Model file for the job. Use its own axes, mm. A direction names the side the tool comes from. Round coordinates to 2 decimals unless told otherwise and drop trailing zeros. Write each loop counter-clockwise with the first axis right and the second up, starting at its lowest first coordinate (ties: lowest second). Pieces come first, ordered by that corner, then holes. Notation, with made-up numbers: (39.5, 61.5) - (98.5, 61.5) arc R27 cw to (98.5, 94.5) - close; hole circle Ø2 at (-12, 11). An arc over 180 degrees is marked (long way). One line per item, written item: value.
from build123d import *

# Parameters (mm, degrees)
SKETCH1_W           = 25
SKETCH1_H           = 25
BOSS_EXTRUDE1_DEPTH = 6
BOSS_EXTRUDE3_DEPTH = 4
SKETCH2_R           = 2.25
CUT_EXTRUDE1_DEPTH  = 6
SKETCH9_W           = 25
SKETCH9_H           = 6
CUT_EXTRUDE2_DEPTH  = 1
SKETCH11_W          = 36.82832664
SKETCH11_H          = 4
BOSS_EXTRUDE4_DEPTH = 20
SKETCH13_R          = 2.1
CUT_EXTRUDE3_DEPTH  = 50.410927182
FILLET2_R           = 10
CHAMFER1_SIZE       = 0.75
CHAMFER2_SIZE       = 0.75
CHAMFER3_SIZE       = 0.75


with BuildPart() as part:
    # Sketch1 → Boss-Extrude1 (new body)
    with BuildSketch(Plane(origin=(0, 0, 0), x_dir=(1, 0, 0), z_dir=(0, 1, 0))):
        with Locations((12.5, 12.5)):
            Rectangle(SKETCH1_W, SKETCH1_H)
    extrude(amount=BOSS_EXTRUDE1_DEPTH)

    # Sketch5 → Boss-Extrude3 (add)
    with BuildSketch(Plane.XY):
        Polygon((-5.91332664, 12.95), (30.915, 12.95), (30, -5.62), (-5, -5.62), align=None)
    extrude(amount=-BOSS_EXTRUDE3_DEPTH)

    # Sketch2 → Cut-Extrude1 (cut)
    with BuildSketch(Plane.XZ):
        with Locations(Location((5.5, -16, 0), (0, 0, 270))):
            Circle(SKETCH2_R)
        with Locations(Location((19.5, -16, 0), (0, 0, 90))):
            Circle(SKETCH2_R)
    extrude(amount=-CUT_EXTRUDE1_DEPTH, mode=Mode.SUBTRACT)

    # Sketch9 → Cut-Extrude2 (cut)
    with BuildSketch(Plane(origin=(0, 0, -25), x_dir=(-1, 0, 0), z_dir=(0, 0, -1))):
        with Locations((-12.5, 3)):
            Rectangle(SKETCH9_W, SKETCH9_H)
    extrude(amount=-CUT_EXTRUDE2_DEPTH, mode=Mode.SUBTRACT)

    # Sketch11 → Boss-Extrude4 (add)
    with BuildSketch(Plane(origin=(0, 12.95, 0), x_dir=(1, 0, 0), z_dir=(0, 1, 0))):
        with Locations((12.50083668, 2)):
            Rectangle(SKETCH11_W, SKETCH11_H)
    extrude(amount=BOSS_EXTRUDE4_DEPTH)

    # Sketch13 → Cut-Extrude3 (cut, through all)
    with BuildSketch(Plane(origin=(0, 0, -4), x_dir=(-1, 0, 0), z_dir=(0, 0, -1))):
        with Locations((-21.25, 26)):
            Circle(SKETCH13_R)
        with Locations((-3.75, 26)):
            Circle(SKETCH13_R)
    extrude(amount=-CUT_EXTRUDE3_DEPTH, mode=Mode.SUBTRACT)

    # Fillet2
    fillet2_edges = [part.edges().sort_by_distance(p)[0] for p in [
        (30, -5.62, -2),
        (-5, -5.62, -2),
        (-5.91332664, 32.95, -2),
        (30.915, 32.95, -2),
    ]]
    fillet(fillet2_edges, radius=FILLET2_R)

    # Chamfer1
    # the kernel refuses this chamfer: 0.75 mm, written as the material it takes off along each edge
    with BuildSketch(Plane(origin=(20.480598416, -5.62, 0), x_dir=(0, 0.9996219169112968, 0.02749587661058636), z_dir=(-1, 0, 0)), Plane(origin=(20.480598416, -5.62, -4), x_dir=(0, -0.02749587661058678, 0.9996219169112968), z_dir=(-1, 0, 0))) as chamfer1_piece_1:
        Polygon((CHAMFER1_SIZE * 0.999621916911, CHAMFER1_SIZE * 0.0274958766106), (-CHAMFER1_SIZE * 0.0274958766106, CHAMFER1_SIZE * 0.999621916911), (0, 0), align=None)
    extrude(amount=15.960340029, mode=Mode.SUBTRACT)
    with BuildSketch(Plane(origin=(31.009920786, 14.876425142, 0), x_dir=(-0.9984106656617833, 0.04919470969738991, 0.027495876610586206), z_dir=(-0.04921331642006734, -0.9987882906236629, 0)), Plane(origin=(31.009920786, 14.876425142, -4), x_dir=(0.027462559599087527, -0.0013531632758839558, 0.9996219169112968), z_dir=(-0.04921331642006734, -0.9987882906236629, 0))) as chamfer1_piece_2:
        Polygon((CHAMFER1_SIZE * 0.999621916911, CHAMFER1_SIZE * 0.0274958766106), (-CHAMFER1_SIZE * 0.0274958766106, CHAMFER1_SIZE * 0.999621916911), (0, 0), align=None)
    extrude(amount=11.001889398, mode=Mode.SUBTRACT)
    with BuildSketch(Plane(origin=(30.915, 11.021237759, 0), x_dir=(-0.9996219169112968, 0, 0.02749587661058636), z_dir=(0, 1, 0)), Plane(origin=(30.915, 11.021237759, -4), x_dir=(0.02749587661058678, 0, 0.9996219169112968), z_dir=(0, 1, 0))) as chamfer1_piece_3:
        Polygon((CHAMFER1_SIZE * 0.999621916911, -CHAMFER1_SIZE * 0.0274958766106), (-CHAMFER1_SIZE * 0.0274958766106, -CHAMFER1_SIZE * 0.999621916911), (0, 0), align=None)
    extrude(amount=11.928762241, mode=Mode.SUBTRACT)
    with BuildSketch(Plane(origin=(4.08667336, 32.95, 0), x_dir=(0, -0.9996219169112968, 0.027495876610586487), z_dir=(1, 0, 0))) as chamfer1_piece_4:
        Polygon((CHAMFER1_SIZE * 0.999621916911, CHAMFER1_SIZE * 0.0274958766106), (-CHAMFER1_SIZE * 0.0274958766106, CHAMFER1_SIZE * 0.999621916911), (0, 0), align=None)
    extrude(amount=16.82832664, mode=Mode.SUBTRACT)
    with BuildSketch(Plane(origin=(-5.91332664, 11.021237759, 0), x_dir=(0.9996219169112968, 0, 0.02749587661058636), z_dir=(0, 1, 0)), Plane(origin=(-5.91332664, 11.021237759, -4), x_dir=(-0.02749587661058678, 0, 0.9996219169112968), z_dir=(0, 1, 0))) as chamfer1_piece_5:
        Polygon((CHAMFER1_SIZE * 0.999621916911, CHAMFER1_SIZE * 0.0274958766106), (-CHAMFER1_SIZE * 0.0274958766106, CHAMFER1_SIZE * 0.999621916911), (0, 0), align=None)
    extrude(amount=11.928762241, mode=Mode.SUBTRACT)
    with BuildSketch(Plane(origin=(20.915, 22.95, 0), x_dir=(1, 0, 0), z_dir=(0, -1, 0))) as chamfer1_piece_6:
        Polygon((10 - CHAMFER1_SIZE, 0), (10, -CHAMFER1_SIZE), (10, 0), align=None)
    revolve(axis=Axis((20.915, 22.95, 0), (0, 0, 1)), revolution_arc=90, mode=Mode.SUBTRACT)
    with BuildSketch(Plane(origin=(4.08667336, 22.95, 0), x_dir=(0, 1, 0), z_dir=(1, 0, 0))) as chamfer1_piece_7:
        Polygon((10 - CHAMFER1_SIZE, 0), (10, -CHAMFER1_SIZE), (10, 0), align=None)
    revolve(axis=Axis((4.08667336, 22.95, 0), (0, 0, 1)), revolution_arc=90, mode=Mode.SUBTRACT)
    with BuildSketch(Plane(origin=(4.520258387, 4.38, 0), x_dir=(0, -1, 0), z_dir=(1, 0, 0))) as chamfer1_piece_8:
        Polygon((10 - CHAMFER1_SIZE, 0), (10, CHAMFER1_SIZE), (10, 0), align=None)
    revolve(axis=Axis((4.520258387, 4.38, 0), (0, 0, -1)), revolution_arc=87.184295724, mode=Mode.SUBTRACT)
    with BuildSketch(Plane(origin=(20.480598416, 4.38, 0), x_dir=(0.9987882906236628, -0.04921331642006739, 0), z_dir=(0.04921331642006739, 0.9987882906236628, 0))) as chamfer1_piece_9:
        Polygon((10 - CHAMFER1_SIZE, 0), (10, CHAMFER1_SIZE), (10, 0), align=None)
    revolve(axis=Axis((20.480598416, 4.38, 0), (0, 0, -1)), revolution_arc=87.179145229, mode=Mode.SUBTRACT)
    with BuildSketch(Plane(origin=(20.915, 32.95, -4), x_dir=(0, 0.02749587661058218, 0.9996219169112969), z_dir=(-1, 0, 0))) as chamfer1_piece_10:
        Polygon((CHAMFER1_SIZE * 0.999621916911, -CHAMFER1_SIZE * 0.0274958766106), (-CHAMFER1_SIZE * 0.0274958766106, -CHAMFER1_SIZE * 0.999621916911), (0, 0), align=None)
    extrude(amount=16.82832664, mode=Mode.SUBTRACT)
    with BuildSketch(Plane(origin=(20.915, 22.95, -4), x_dir=(1, 0, 0), z_dir=(0, -1, 0))) as chamfer1_piece_11:
        Polygon((10, CHAMFER1_SIZE), (10 - CHAMFER1_SIZE, 0), (10, 0), align=None)
    revolve(axis=Axis((20.915, 22.95, -4), (0, 0, 1)), revolution_arc=90, mode=Mode.SUBTRACT)
    with BuildSketch(Plane(origin=(4.08667336, 22.95, -4), x_dir=(0, 1, 0), z_dir=(1, 0, 0))) as chamfer1_piece_12:
        Polygon((10, CHAMFER1_SIZE), (10 - CHAMFER1_SIZE, 0), (10, 0), align=None)
    revolve(axis=Axis((4.08667336, 22.95, -4), (0, 0, 1)), revolution_arc=90, mode=Mode.SUBTRACT)
    with BuildSketch(Plane(origin=(4.520258387, 4.38, -4), x_dir=(0, -1, 0), z_dir=(1, 0, 0))) as chamfer1_piece_13:
        Polygon((10, -CHAMFER1_SIZE), (10 - CHAMFER1_SIZE, 0), (10, 0), align=None)
    revolve(axis=Axis((4.520258387, 4.38, -4), (0, 0, -1)), revolution_arc=87.184295724, mode=Mode.SUBTRACT)
    with BuildSketch(Plane(origin=(20.480598416, 4.38, -4), x_dir=(0.9987882906236628, -0.04921331642006739, 0), z_dir=(0.04921331642006739, 0.9987882906236628, 0))) as chamfer1_piece_14:
        Polygon((10, -CHAMFER1_SIZE), (10 - CHAMFER1_SIZE, 0), (10, 0), align=None)
    revolve(axis=Axis((20.480598416, 4.38, -4), (0, 0, -1)), revolution_arc=87.179145229, mode=Mode.SUBTRACT)
    with BuildSketch(Plane(origin=(-5.467668718, 3.888764679, 0), x_dir=(0.998415083892051, 0.049104959283599446, 0.027495876610586386), z_dir=(-0.04912353206032882, 0.9987927105250207, 0)), Plane(origin=(-5.467668718, 3.888764679, -4), x_dir=(-0.02746268112814937, -0.0013506945762069992, 0.9996219169112968), z_dir=(-0.04912353206032882, 0.9987927105250207, 0))) as chamfer1_piece_15:
        Polygon((CHAMFER1_SIZE * 0.999621916911, CHAMFER1_SIZE * 0.0274958766106), (-CHAMFER1_SIZE * 0.0274958766106, CHAMFER1_SIZE * 0.999621916911), (0, 0), align=None)
    extrude(amount=11.000950319, mode=Mode.SUBTRACT)
    with BuildSketch(Plane(origin=(21.25, 26, 0), x_dir=(-1, 0, 0), z_dir=(0, -1, 0))) as chamfer1_piece_16:
        Polygon((2.1 + CHAMFER1_SIZE, 0), (2.1, CHAMFER1_SIZE), (2.1, 0), align=None)
    revolve(axis=Axis((21.25, 26, 0), (0, 0, -1)), mode=Mode.SUBTRACT)
    with BuildSketch(Plane(origin=(21.25, 26, -4), x_dir=(-1, 0, 0), z_dir=(0, -1, 0))) as chamfer1_piece_17:
        Polygon((2.1, -CHAMFER1_SIZE), (2.1 + CHAMFER1_SIZE, 0), (2.1, 0), align=None)
    revolve(axis=Axis((21.25, 26, -4), (0, 0, -1)), mode=Mode.SUBTRACT)
    with BuildSketch(Plane(origin=(3.75, 26, 0), x_dir=(-1, 0, 0), z_dir=(0, -1, 0))) as chamfer1_piece_18:
        Polygon((2.1 + CHAMFER1_SIZE, 0), (2.1, CHAMFER1_SIZE), (2.1, 0), align=None)
    revolve(axis=Axis((3.75, 26, 0), (0, 0, -1)), mode=Mode.SUBTRACT)
    with BuildSketch(Plane(origin=(3.75, 26, -4), x_dir=(-1, 0, 0), z_dir=(0, -1, 0))) as chamfer1_piece_19:
        Polygon((2.1, -CHAMFER1_SIZE), (2.1 + CHAMFER1_SIZE, 0), (2.1, 0), align=None)
    revolve(axis=Axis((3.75, 26, -4), (0, 0, -1)), mode=Mode.SUBTRACT)

    # Chamfer2
    chamfer2_edges = [part.edges().sort_by_distance(p)[0] for p in [
        (5.5, 6, -13.75),
        (5.5, 0, -13.75),
        (19.5, 6, -18.25),
        (19.5, 0, -18.25),
    ]]
    chamfer(chamfer2_edges, length=CHAMFER2_SIZE)

    # Chamfer3
    chamfer3_edges = [part.edges().sort_by_distance(p)[0] for p in [
        (25, 0, -14),
        (25, 6, -14),
        (0, 0, -14),
        (0, 6, -14),
        (25, 3, -24),
        (12.5, 6, -24),
        (0, 3, -24),
        (12.5, 0, -24),
    ]]
    chamfer(chamfer3_edges, length=CHAMFER3_SIZE)


solid = part.part
1. Band-saw the part on D-D on y = 26. State how many separate pieces and enclosed holes the cut face has, plus the area to 3 significant figures.
Report:
separate pieces: 3
enclosed holes: 0
area: 106 mm²
2. Drop flat-ended pins along their axis: pin 1 (2.5 mm diameter, centred on x = 19.5, z = -16, fed in from +Y); pin 2 (3 mm diameter, centred on x = 10.5, z = -12.5, fed in from +Y); pin 3 (5 mm diameter, centred on y = 3, z = -12, fed in from -X); pin 4 (5 mm diameter, centred on x = 3.75, y = 26, fed in from -Z). Give the stop position or say it passes through.
Report:
pin 1: through
pin 2: y = 6
pin 3: x = 0
pin 4: z = -3.65
3. Band-saw the part on B-B on z = -7. Write the cut outline in (x, y), plus the area to 3 significant figures.
Report:
outline: (0, 0.75) - (0.75, 0) - (24.25, 0) - (25, 0.75) - (25, 5.25) - (24.25, 6) - (0.75, 6) - (0, 5.25) - close
area: 149 mm²
4. Tool access for faces 1 (the face through (27.298, -2.936, -2.018)), 2 (the face through (12, 0, -14)), 3 (the face through (0, 3, -13)), 4 (the face through (25, 3, -13)): list every direction of +Z, -Z, +X, -X, +Y, -Y with a clear straight run to the whole face (end or side of a thin tool).
Report:
face 1: +Z, -Z, +X, -Y
face 2: -Z, +X, -X, -Y
face 3: -Z, -X, +Y, -Y
face 4: -Z, +X, +Y, -Y
5. Band-saw the part on C-C on y = 7.5. Write the cut outline in (x, z), plus the area to 3 significant figures.
Report:
outline: (-5.65, -3.25) - (-4.89, -4) - (29.9, -4) - (30.65, -3.25) - (30.65, -0.75) - (29.9, 0) - (-4.89, 0) - (-5.65, -0.75) - close
area: 144 mm²
6. Wall check: probe 1 along X at (y, z) = (1.7, -16); probe 2 along Z at (x, y) = (19.5, 3.25); probe 3 along Z at (x, y) = (16, 28). Give the ranges that are in metal, low to high. Write a range as [from, to].
Report:
probe 1: [0, 3.25], [7.75, 17.25], [21.75, 25]
probe 2: [-24, -18.25], [-13.75, 0]
probe 3: [-4, 0]
7. Band-saw the part on A-A on z = -16. Write the cut outline in (x, y), plus the area to 3 significant figures.
Report:
outline: (0, 0.75) - (0.75, 0) - (2.5, 0) - (3.25, 0.75) - (3.25, 5.25) - (2.5, 6) - (0.75, 6) - (0, 5.25) - close; (7.75, 0.75) - (8.5, 0) - (16.5, 0) - (17.25, 0.75) - (17.25, 5.25) - (16.5, 6) - (8.5, 6) - (7.75, 5.25) - close; (21.75, 0.75) - (22.5, 0) - (24.25, 0) - (25, 0.75) - (25, 5.25) - (24.25, 6) - (22.5, 6) - (21.75, 5.25) - close
area: 92.6 mm²
